Part model, mm, in its own coordinate system. A direction names the side the tool comes from. Coordinates: 2 decimals unless noted, no trailing zeros. Write each loop counter-clockwise with the first axis right and the second up, starting at its lowest first coordinate (ties: lowest second). Pieces come first, ordered by that corner, then holes. Notation, with made-up numbers: (-15.5, 0) -> (37.5, 0) arc R21 ccw to (37.5, 36) -> close; hole circle Ø8 at (20, 57.25). An arc over 180 degrees is marked (long way). Write item = value, one per line.
from build123d import *

# Parameters (mm, degrees)
EXTRUDE_1_DEPTH     = 25
SKETCH_2_W          = 53
SKETCH_2_H          = 49
EXTRUDE_2_DEPTH     = 11
SKETCH_4_R          = 2.75
CUT_EXTRUDE_1_DEPTH = 2
SKETCH_5_R          = 1.75
CUT_EXTRUDE_2_DEPTH = 76.193084788
SKETCH_8_W          = 33
SKETCH_8_H          = 3.5
CUT_EXTRUDE_3_DEPTH = 77.387171698
EXTRUDE_3_DEPTH     = 10


with BuildPart() as part:
    # 草图1 → 凸台-拉伸1 (new body)
    with BuildSketch(Plane.XY):
        Polygon((0, 43), (0, 46), (-53, 46), (-53, -3), (0, -3), (0, 0), (-50, 0), (-50, 43), align=None)
    extrude(amount=EXTRUDE_1_DEPTH)

    # 草图2 → 凸台-拉伸2 (add)
    with BuildSketch(Plane(origin=(0, 0, 0), x_dir=(-1, 0, 0), z_dir=(0, 0, -1))):
        with Locations((26.5, 21.5)):
            Rectangle(SKETCH_2_W, SKETCH_2_H)
    extrude(amount=EXTRUDE_2_DEPTH)

    # 草图4 → 切除-拉伸1 (cut)
    with BuildSketch(Plane.XY):
        with Locations((-26, 35)):
            Circle(SKETCH_4_R)
        with Locations((-26, 8)):
            Circle(SKETCH_4_R)
    extrude(amount=-CUT_EXTRUDE_1_DEPTH, mode=Mode.SUBTRACT)

    # 草图5 → 切除-拉伸2 (cut, through all)
    with BuildSketch(Plane.XY.offset(-2)):
        with Locations((-26, 8)):
            Circle(SKETCH_5_R)
        with Locations((-26, 35)):
            Circle(SKETCH_5_R)
    extrude(amount=-CUT_EXTRUDE_2_DEPTH, mode=Mode.SUBTRACT)

    # 草图8 → 切除-拉伸3 (cut, through all)
    with BuildSketch(Plane.XZ.offset(3)):
        with Locations((-21.5, -6.25)):
            Rectangle(SKETCH_8_W, SKETCH_8_H)
    extrude(amount=-CUT_EXTRUDE_3_DEPTH, mode=Mode.SUBTRACT)

    # 草图9 → 凸台-拉伸3 (add)
    with BuildSketch(Plane(origin=(0, 0, 0), x_dir=(0, 0, -1), z_dir=(1, 0, 0))):
        Polygon((-25, 43), (0, 43), (0, 0), (-25, 0), (-25, -3), (11, -3), (11, 46), (-25, 46), align=None)
    extrude(amount=EXTRUDE_3_DEPTH)


solid = part.part
Q1. Saw through at A-A on y = 8. Give the cut face in (x, z), and give its area (3 significant figures).
Model answer:
outline = (-53, -11) -> (-27.75, -11) -> (-27.75, -8) -> (-38, -8) -> (-38, -4.5) -> (-27.75, -4.5) -> (-27.75, -2) -> (-28.75, -2) -> (-28.75, 0) -> (-50, 0) -> (-50, 25) -> (-53, 25) -> close; (-24.25, -11) -> (10, -11) -> (10, 0) -> (-23.25, 0) -> (-23.25, -2) -> (-24.25, -2) -> (-24.25, -4.5) -> (-5, -4.5) -> (-5, -8) -> (-24.25, -8) -> close
area = 622 mm²
Q2. Saw through at B-B on x = -10.5. Give the cut face in (y, z), and give its area (4 significant figures).
Model answer:
outline = (-3, -11) -> (46, -11) -> (46, -8) -> (-3, -8) -> close; (-3, -4.5) -> (46, -4.5) -> (46, 25) -> (43, 25) -> (43, 0) -> (0, 0) -> (0, 25) -> (-3, 25) -> close
area = 517.5 mm²
Q3. Saw through at C-C on y = 22. Give the cut face in (x, z), and give its area (4 significant figures).
Model answer:
outline = (-53, -11) -> (10, -11) -> (10, 0) -> (-50, 0) -> (-50, 25) -> (-53, 25) -> close; hole (-38, -8) -> (-5, -8) -> (-5, -4.5) -> (-38, -4.5) -> close
area = 652.5 mm²
Q4. Mould opens along Y. For faces 6 (the face through (-22, 46, 7)), 7 (the face through (-20, 43, 13)), 8 (the face through (10, 27, -1)) say: released by +Y, released by -Y, zero draft, split by the parting line, or undercut.
Model answer:
face_6 = released by +Y
face_7 = undercut
face_8 = zero draft
Q5. Which spindle directions (+Z, -Z, +X, -X, +Y, -Y) get a long thin tool onto all of the face, cutting with end or side? Do faces 1 (the face through (-38, 21, -6)), 2 (the face through (-26.3, 43.4, 25)), 3 (the face through (-27.75, 8.08, -9.48)), 4 (the face through (-20, 22, 0)), 5 (the face through (-26, 6, -2)). Say none if no direction does.
Model answer:
face_1 = +Y, -Y
face_2 = +Z, +X, -X, +Y, -Y
face_3 = +Z, -Z
face_4 = +Z, +X
face_5 = +Z
Q6. Pin check, flat tips, straight feed: pin 1 (10 mm diameter, centred on y = 24, z = 19, fed in from +X); pin 2 (10 mm diameter, centred on x = -7, z = -6.5, fed in from +Y); pin 3 (4.5 mm diameter, centred on x = -26, y = 8, fed in from +Z); pin 4 (16.5 mm diameter, centred on x = -23, y = 17, fed in from +Z). Stop position of each tip, or through.
Model answer:
pin_1 = -50
pin_2 = 46
pin_3 = -2
pin_4 = 0
Q7. Probe line 1 (Y direction, x = -26, z = -3.15); line 2 (Y direction, x = -32, z = 7); line 3 (Z direction, x = -32, y = 3). List the from-to ranges inside material, lowest first. Write a range as from..to.
Model answer:
line_1 = -3..6.25, 9.75..33.25, 36.75..46
line_2 = -3..0, 43..46
line_3 = -11..-8, -4.5..0
Q8. Saw through at D-D on z = 13. Give the cut face in (x, y).
Model answer:
outline = (-53, -3) -> (10, -3) -> (10, 0) -> (-50, 0) -> (-50, 43) -> (10, 43) -> (10, 46) -> (-53, 46) -> close
